Can you work these out from the drawing? Everything is in mm from the part's minimum corner. Round coordinates to 2 decimals unless told otherwise and drop trailing zeros. Loops run counter-clockwise (first coordinate to the right, second up) from the corner with the lowest first, then second, coordinate; pieces in that order, holes last. Notation, with made-up numbers: (47.25, -20) - (52.25, -20) arc R33 ccw to (52.25, 18) - close; hole circle Ø8 at (63, 88). An arc over 180 degrees is marked (long way). Put each result on its own line as item: value. Start each with the question number.
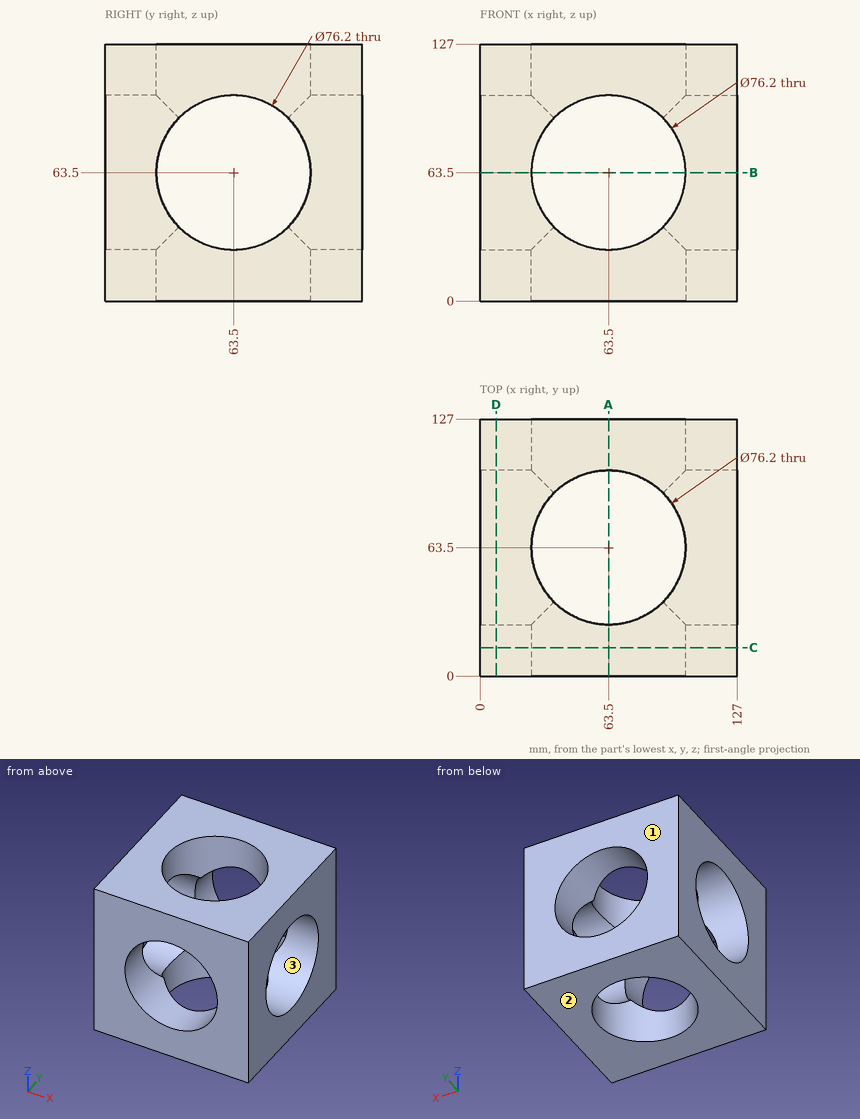
Item 1: Suppose I cut it at C-C, the plane y = 14. List the corners of the cut face in (x, z) for me, then the cut area to 3 significant figures.
Item 2: Suppose I cut it at A-A, the plane x = 63.5. List the corners of the cut face in (y, z) for me.
Item 3: I need wall thicknesses on line 1 (Z direction, x = 19.5, y = 63.5). Which ranges of the line are inside material? Lowest first, please. Write a range as from..to.
Item 4: Thinking about a two-plate mould opening in Y: for the marked faces 1, 2 and 3, which applies, released by +Y, released by -Y, zero draft, split by the parting line, or undercut?
Numbers:
1. outline: (0, 0) - (127, 0) - (127, 127) - (0, 127) - close; hole circle Ø76.2 at (63.5, 63.5)
1. area: 11,600 mm^2
2. outline: (0, 0) - (25.4, 0) - (25.4, 25.4) - (0, 25.4) - close; (0, 101.6) - (25.4, 101.6) - (25.4, 127) - (0, 127) - close; (101.6, 0) - (127, 0) - (127, 25.4) - (101.6, 25.4) - close; (101.6, 101.6) - (127, 101.6) - (127, 127) - (101.6, 127) - close
3. line 1: 0..25.4, 101.6..127
4. face 1: released by +Y
4. face 2: zero draft
4. face 3: undercut
